CAD build for the part. Positions are in the model's coordinates, mm. Coordinates: 2 decimals unless noted, no trailing zeros. Order: outer loops, then holes, each group sorted by start corner. A loop starts at its lowest first (then second) coordinate and runs counter-clockwise, first axis right, second up. Notation, with made-up numbers: M 31,0.25 L 38,0.25 A21 cw 38,29.25 Z; hole C 32,89 d1. An arc over 180 degrees is marked long. Write item = value, one per line. Start each with the question number.
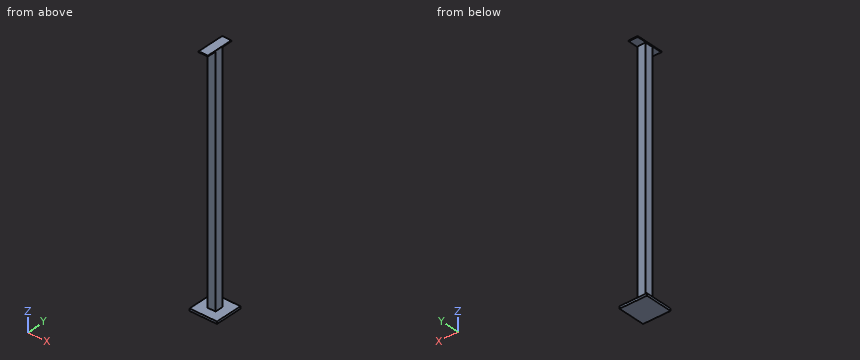
```python
from build123d import *

# Parameters (mm, degrees)
F0_W     = 300
F0_H     = 300
F0_W_2   = 90
F0_H_2   = 90
F1_DEPTH = 25
F2_DEPTH = 2600
F3_W     = 100
F3_H     = 300
F4_DEPTH = 10


with BuildPart() as f1:
    # F0 (on Top) → F1 (new body)
    with BuildSketch(Plane.XY):
        with Locations((150, 150)):
            Rectangle(F0_W, F0_H)
        with Locations((150, 150)):
            Rectangle(F0_W_2, F0_H_2, mode=Mode.SUBTRACT)
        with Locations((150, 150)):
            Rectangle(F0_W_2, F0_H_2)
    extrude(amount=-F1_DEPTH)

    # F0 (on Top) → F2 (join)
    with BuildSketch(Plane.XY):
        with Locations((150, 150)):
            Rectangle(F0_W_2, F0_H_2)
    extrude(amount=F2_DEPTH)

    # F3 (on face) → F4 (join)
    with BuildSketch(Plane.XY.offset(2600)):
        with Locations((150, 150)):
            Rectangle(F3_W, F3_H)
    extrude(amount=F4_DEPTH)


solid = f1.part
```
1. Slice it at B-B (x = 171.5). Write the cut outline in (y, z), plus the area to 4 significant figures.
2. Probe L1, parallel to Z at x = 143, y = 13; L2, parallel to Z at x = 56, y = 57; L3, parallel to Y at x = 190.5, z = 1557.5. List the from-to ranges inside material, lowest first.
3. Slice it at A-A (y = 255.5). Write the cut outline in (x, z), plus the area to 3 significant figures.
4. Flat gauge pins, fed straight in: pin 1 (3 mm diameter, centred on x = 189, z = 1788, fed in from -Y); pin 2 (1 mm diameter, centred on y = 123, z = 412, fed in from -X); pin 3 (8 mm diameter, centred on x = 107, z = 2061, fed in from +Y). Where does each tip first touch, or does it go through?
5. Slice it at C-C (z = 1288). Write the cut outline in (x, y), plus the area to 3 significant figures.
Calculated:
q1.outline = M 0,-25 L 300,-25 L 300,0 L 195,0 L 195,2600 L 300,2600 L 300,2610 L 0,2610 L 0,2600 L 105,2600 L 105,0 L 0,0 Z
q1.area = 244,500 mm²
q2.L1 = -25 to 0, 2600 to 2610
q2.L2 = -25 to 0
q2.L3 = 105 to 195
q3.outline = M 0,-25 L 300,-25 L 300,0 L 0,0 Z; M 100,2600 L 200,2600 L 200,2610 L 100,2610 Z
q3.area = 8,500 mm²
q4.pin_1 = 105
q4.pin_2 = 105
q4.pin_3 = 195
q5.outline = M 105,105 L 195,105 L 195,195 L 105,195 Z
q5.area = 8,100 mm²
